For this review, take the finished solid that the model builds, in its own axes (mm). Give positions to 0.01 mm unless a question says otherwise; leave off trailing zeros. Write each loop counter-clockwise with the first axis right and the second up, starting at its lowest first coordinate (ties: lowest second). Pieces come first, ordered by that corner, then holes. Notation, with made-up numbers: M -1.75,-8 L 7.25,-8 A20 ccw 7.25,0 Z; hole C 8.5,35.25 d11. An arc over 180 degrees is marked long. Write item = value, one per line.
```python
from build123d import *
from OCP.BRepFilletAPI import BRepFilletAPI_MakeChamfer

# Parameters (mm, degrees)
SZKIC1_W                   = 4.712
SZKIC1_H                   = 9.3
SFAZOWANIE1_SIZE           = 1.2
SFAZOWANIE1_SIZE2          = 0.692820323
SZKIC2_OUTSIDE_W           = 25.168
SZKIC2_OUTSIDE_H           = 25.168
WYTNIJ_WYCI_GNI_CIE1_DEPTH = 16.649600634


with BuildPart() as part:
    # Szkic1 → Obrót1 (revolve)
    with BuildSketch(Plane.XY, mode=Mode.PRIVATE) as obr_t1_sk:
        with Locations((6.544, 4.65)):
            Rectangle(SZKIC1_W, SZKIC1_H)
    revolve(obr_t1_sk.sketch.rotate(Axis((0, 0, 0), (0, 1, 0)), 90), axis=Axis((0, 0, 0), (0, 1, 0)))

    # Sfazowanie1: one chamfer whose edges measure the first distance from different faces: ONE call of the kernel's chamfer builder (chamfer() names one face for all edges)
    sfazowanie1_edges_1 = [part.edges().sort_by_distance(p)[0] for p in [
        (0, 0, 8.9),
    ]]
    sfazowanie1_side_1 = [part.faces().sort_by_distance(p)[0] for p in [
        (0, 0, 4.439730014),
    ]]
    sfazowanie1_edges_2 = [part.edges().sort_by_distance(p)[0] for p in [
        (0, 9.3, 8.9),
    ]]
    sfazowanie1_side_2 = [part.faces().sort_by_distance(p)[0] for p in [
        (0, 9.3, 8.648269986),
    ]]
    sfazowanie1 = BRepFilletAPI_MakeChamfer(part.part.solid().wrapped)
    for e in sfazowanie1_edges_1:
        sfazowanie1.Add(SFAZOWANIE1_SIZE, SFAZOWANIE1_SIZE2, e.wrapped, sfazowanie1_side_1[0].wrapped)  # the first distance lies on this face
    for e in sfazowanie1_edges_2:
        sfazowanie1.Add(SFAZOWANIE1_SIZE, SFAZOWANIE1_SIZE2, e.wrapped, sfazowanie1_side_2[0].wrapped)  # the first distance lies on this face
    add(Compound.cast(sfazowanie1.Shape()), mode=Mode.REPLACE)

    # Szkic2 outside → Wytnij-wyciągnięcie1 (cut, through all)
    with BuildSketch(Plane(origin=(0, 9.3, 0), x_dir=(1, 0, 0), z_dir=(0, 1, 0))):
        Rectangle(SZKIC2_OUTSIDE_W, SZKIC2_OUTSIDE_H)
        Polygon((7.707626094, 4.45), (0, 8.9), (-7.707626094, 4.45), (-7.707626094, -4.45), (0, -8.9), (7.707626094, -4.45), align=None, mode=Mode.SUBTRACT)
    extrude(amount=-WYTNIJ_WYCI_GNI_CIE1_DEPTH, mode=Mode.SUBTRACT)


solid = part.part
```
1. For line 1 along X through (y, z) = (7.75, 0); line 2 along Z through (x, y) = (-1.75, 1.25); line 3 along X through (y, z) = (4.25, -2.75), list the stretches that pass through material, from the lowest coordinate up. Write a range as from..to.
Responses:
line_1 = -7.71..-4.19, 4.19..7.71
line_2 = -7.89..-3.8, 3.8..7.89
line_3 = -7.71..-3.16, 3.16..7.71
2. The part is to be moulded in two halves that separate along X. For faces 1 (the face through (7.708, 5, 0)), 2 (the face through (-3.8, 4.715, -6.706)), 3 (the face through (3.3, 0, 3.3)), 4 (the face through (-0.184, 4.715, 4.184)), say which applies: +X half, -X half, draft (parallel to the pull), parting line (faces both ways), or undercut.
Responses:
face_1 = +X half
face_2 = -X half
face_3 = draft
face_4 = undercut
3. Insertion check: P1, Ø3, axis at x = 2, y = 7, coming from the +Z side. The pin has a flat end and moves straight along its axis. Give the tip position at first contact, or say it passes through.
Responses:
P1 = 8.61
4. We need section B-B, the plane y = 6.5. Write out the cut boundary in (x, z), then the cut area to 3 significant figures.
Responses:
outline = M -7.71,-4.45 L 0,-8.9 L 7.71,-4.45 L 7.71,4.45 L 0,8.9 L -7.71,4.45 Z; hole C 0,0 d8.38
area = 151 mm2
